Design review of the part shown in the three views and the two pictorial views. Dimensions are in mm from the part's minimum x, y and z. Coordinates: 2 decimals unless noted, no trailing zeros. Loops run counter-clockwise (first coordinate to the right, second up) from the corner with the lowest first, then second, coordinate; pieces in that order, holes last. Notation, with made-up numbers: M 49.25,38.25 L 53.25,38.25 A9 cw 53.25,54.25 Z; hole C 64,-7 d10. An arc over 180 degrees is marked long. Put each result on its own line as item: value. Start each with the question number.
(1) Take a section at D-D, the plane x = 6. Give the boundary of the cut face in (y, z).
(2) The part is to be moulded in two halves that separate along Z. For the marked faces 1, 2, 3 and 4, say which applies: +Z half, -Z half, draft (parallel to the pull), parting line (faces both ways), or undercut.
(3) Clearance check with flat-ended pins moving along their axes: pin 1 (1.5 mm diameter, centred on y = 3, z = 8.5, fed in from -X); pin 2 (1.5 mm diameter, centred on y = 2, z = 16.5, fed in from +X). State where each tip first meets the part, or that it passes through.
(4) For probe 1 along Z at (x, y) = (8, 3.2); probe 2 along X at (y, z) = (4.5, 11); probe 3 along Z at (x, y) = (5.5, 2.85), list the stretches that pass through material, from the lowest coordinate up. Write a range as [from, to].
(5) Take a section at C-C, the plane x = 9.5. Give the boundary of the cut face in (y, z), then the cut area to 3 significant figures.
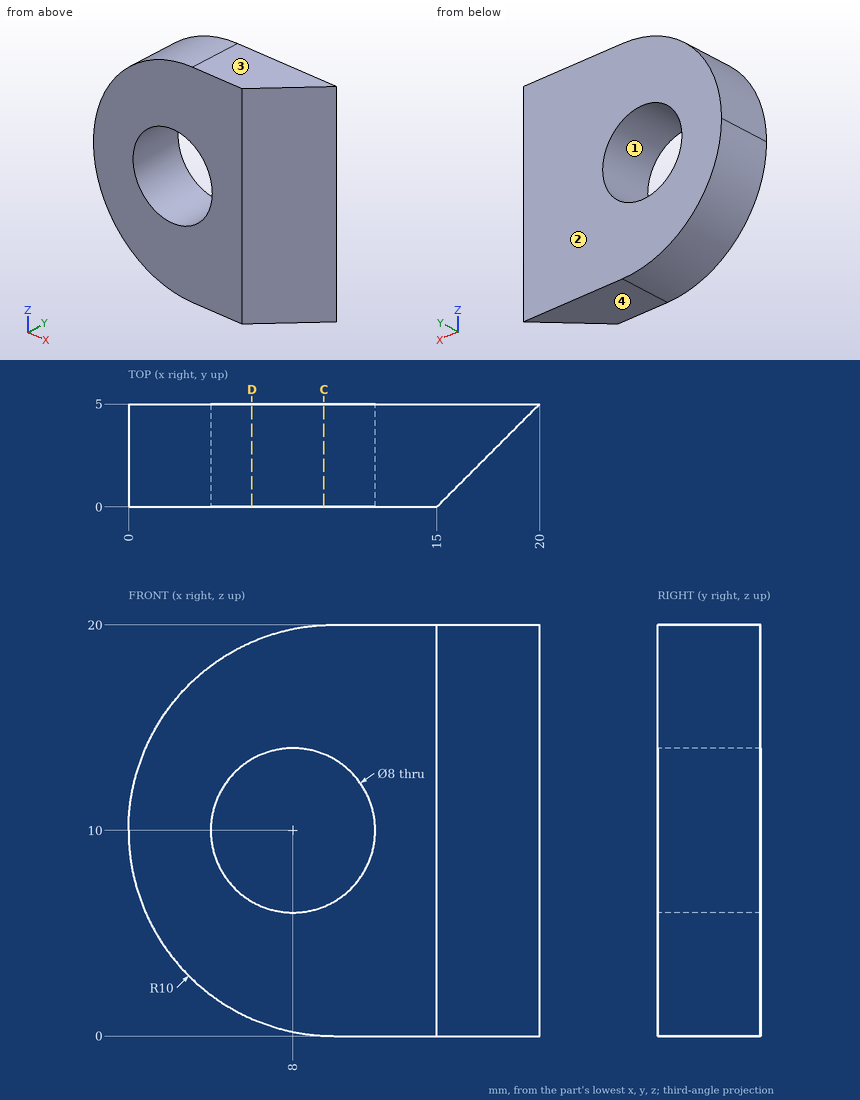
Computed values:
1. outline: M 0,0.83 L 5,0.83 L 5,6.54 L 0,6.54 Z; M 0,13.46 L 5,13.46 L 5,19.17 L 0,19.17 Z
2. face 1: undercut
2. face 2: draft
2. face 3: +Z half
2. face 4: -Z half
3. pin 1: stops at x = 0.03
3. pin 2: stops at x = 17.75
4. probe 1: z = [0.2, 6], [14, 19.8]
4. probe 2: x = [0.05, 4.13], [11.87, 19.5]
4. probe 3: z = [1.07, 6.88], [13.12, 18.93]
5. outline: M 0,0.01 L 5,0.01 L 5,6.29 L 0,6.29 Z; M 0,13.71 L 5,13.71 L 5,19.99 L 0,19.99 Z
5. area: 62.8 mm^2
